Verification items for the finished model (mm, model axes). A direction names the side the tool comes from. Round coordinates to 2 decimals unless told otherwise and drop trailing zeros. Order: outer loops, then holes, each group sorted by start corner. A loop starts at its lowest first (then second) coordinate and runs counter-clockwise, first axis right, second up. Notation, with made-up numbers: (-12, -32) -> (-7, -32) arc R14 ccw to (-7, -20) -> close; hole circle Ø3 at (73.5, 87). An arc over 180 degrees is marked (long way). Return JSON: item names as keys, results as strings. Group by question number.
1) Section check A-A on y = -2.4. State how many separate pieces and enclosed holes the cut face has, plus the area to 3 significant figures.
2) Section check D-D on z = 29. Enter the section's corners in (x, y), plus the area to 3 significant figures.
3) Draft check along Z on faces 5 (the cylindrical face through (-0.065, -1.503, 123.825)), 6 (the flat face through (10, -3.048, 58)), 7 (the flat face through (0, -2, 73)), 8 (the cylindrical face through (-12.038, -1.503, 53.15)). Enter one of: pulls with the +Z half, pulls with the -Z half, needs draft (parallel to the pull), parting line crosses it, or undercut.
4) Section check C-C on z = 51. Enter the section's corners in (x, y), plus the area to 3 significant figures.
5) Scan lines: L1, parallel to Z at x = 44.45, y = -1.05 (3 decimals); L2, parallel to Z at x = -1, y = -1.75; L3, parallel to Z at x = -4.5, y = -1.75. Record each from-to range of solid material in increasing order.
6) Section check B-B on x = -5.5. Enter the section's corners in (y, z), plus the area to 3 significant figures.
7) Depth check by flat-ended pin: pin 1 (5.5 mm diameter, centred on x = 0, z = 114.3, fed in from +Y); pin 2 (1 mm diameter, centred on y = -1.5, z = 98.5, fed in from +X); pin 3 (0.9 mm diameter, centred on y = -2, z = 30, fed in from -X). Enter the tip coordinate at first touch or a pass-through.
8) Tool access check on faces 1 (the flat face through (-0.57, -1.5, 72.92)), 2 (the flat face through (13.134, -1.503, 37.784)), 3 (the flat face through (0, -2, 29)), 4 (the flat face through (10, 0, 58)). Record the directions out of +Z, -Z, +X, -X, +Y, -Y that give a thin tool (end or side, any length) a straight path to the whole face; none if there is none.
```python
from build123d import *

# Parameters (mm, degrees)
F1_DEPTH = 3.048


with BuildPart() as f1:
    # F0 (on Front) → F1 (new body)
    with BuildSketch(Plane.XZ):
        with BuildLine():
            ThreePointArc((15.0989586091, 58.5972381334), (15.6797894265, 61.0180998126), (15.875, 63.5))
            ThreePointArc((15.875, 63.5), (15.843643726, 64.4972855577), (15.7496987737, 65.4906314418))
            Line((15.7496987737, 65.4906314418), (15.0989586091, 58.5972381334))
        make_face()
        with BuildLine():
            Line((15.0989586091, 58.5972381334), (15.7496987737, 65.4906314418))
            ThreePointArc((15.7496987737, 65.4906314418), (10.4979605367, 75.408335298), (0, 79.375))
            Line((0, 79.375), (0, 66.675))
            ThreePointArc((0, 66.675), (2.2450640303, 65.7450640303), (3.175, 63.5))
            ThreePointArc((3.175, 63.5), (2.2450640303, 61.2549359697), (0, 60.325))
            Line((0, 60.325), (0, 47.625))
            ThreePointArc((0, 47.625), (9.3323169783, 50.6577461162), (15.0989586091, 58.5972381334))
        make_face()
        with BuildLine():
            ThreePointArc((0, 79.375), (10.4979605367, 75.408335298), (15.7496987737, 65.4906314418))
            Line((15.7496987737, 65.4906314418), (9.5073556067, 114.8794949239))
            ThreePointArc((9.5073556067, 114.8794949239), (9.5205878798, 114.5898817394), (9.525, 114.3))
            ThreePointArc((9.525, 114.3), (6.7351920908, 107.5648079092), (0, 104.775))
            Line((0, 104.775), (0, 79.375))
        make_face()
        with BuildLine():
            Line((11.2237043258, 17.546057651), (15.0989586091, 58.5972381334))
            ThreePointArc((15.0989586091, 58.5972381334), (9.3323169783, 50.6577461162), (0, 47.625))
            Line((0, 47.625), (0, 9.525))
            ThreePointArc((0, 9.525), (6.7351920908, 6.7351920908), (9.525, 0))
            Line((9.525, 0), (36.5125, 0))
            ThreePointArc((36.5125, 0), (38.9380895153, 5.7116327839), (44.7324052746, 7.9324746146))
            Line((44.7324052746, 7.9324746146), (18.8558582529, 8.853709629))
            ThreePointArc((18.8558582529, 8.853709629), (13.1645636219, 11.5533837704), (11.2237043258, 17.546057651))
        make_face()
        with BuildLine():
            ThreePointArc((-0.9612294652, 79.3458721096), (-0.4808353457, 79.3677163565), (0, 79.375))
            Line((0, 79.375), (0, 104.775))
            ThreePointArc((0, 104.775), (-6.7492648996, 107.5789101839), (-9.5249166577, 114.339845498))
            Line((-9.5249166577, 114.339845498), (-15.7476590945, 65.5067032771))
            ThreePointArc((-15.7476590945, 65.5067032771), (-10.8479208938, 75.0904373205), (-0.9612294652, 79.3458721096))
        make_face()
        with BuildLine():
            ThreePointArc((-0.6240967535, 99.9581825499), (-1.0555795763, 98.8701657595), (-2.1154738069, 98.3735953389))
            ThreePointArc((-2.1154738069, 98.3735953389), (-3.3676139306, 101.0461993403), (-0.6240967535, 99.9581825499))
        make_face(mode=Mode.SUBTRACT)
        with BuildLine():
            ThreePointArc((9.525, 114.3), (9.5205878798, 114.5898817394), (9.5073556067, 114.8794949239))
            ThreePointArc((9.5073556067, 114.8794949239), (-0.2699675413, 123.8211733797), (-9.5249166577, 114.339845498))
            ThreePointArc((-9.5249166577, 114.339845498), (-6.7492648996, 107.5789101839), (0, 104.775))
            ThreePointArc((0, 104.775), (6.7351920908, 107.5648079092), (9.525, 114.3))
        make_face()
        with BuildLine():
            ThreePointArc((3.175, 114.3), (2.2450640303, 112.0549359697), (0, 111.125))
            ThreePointArc((0, 111.125), (-2.2450640303, 116.5450640303), (3.175, 114.3))
        make_face(mode=Mode.SUBTRACT)
        with BuildLine():
            ThreePointArc((-15.0944695401, 58.5834347047), (-9.3264449534, 50.6534810345), (0, 47.625))
            Line((0, 47.625), (0, 60.325))
            ThreePointArc((0, 60.325), (-3.1735432713, 63.4038329309), (-0.192245893, 66.6691744219))
            Line((-0.192245893, 66.6691744219), (-0.9612294652, 79.3458721096))
            ThreePointArc((-0.9612294652, 79.3458721096), (-10.8479208938, 75.0904373205), (-15.7476590945, 65.5067032771))
            Line((-15.7476590945, 65.5067032771), (-15.0944695401, 58.5834347047))
        make_face()
        with BuildLine():
            ThreePointArc((-15.7476590945, 65.5067032771), (-15.8048137164, 62.00886339), (-15.0944695401, 58.5834347047))
            Line((-15.0944695401, 58.5834347047), (-15.7476590945, 65.5067032771))
        make_face()
        with BuildLine():
            ThreePointArc((9.525, 0), (6.7351920908, 6.7351920908), (0, 9.525))
            Line((0, 9.525), (0, 3.175))
            ThreePointArc((0, 3.175), (2.2450640303, 2.2450640303), (3.175, 0))
            Line((3.175, 0), (9.525, 0))
        make_face()
        with BuildLine():
            Line((0, 3.175), (0, 9.525))
            ThreePointArc((0, 9.525), (-9.525, 0), (0, -9.525))
            Line((0, -9.525), (0.6773435479, -9.500885786))
            ThreePointArc((0.6773435479, -9.500885786), (6.9705567315, -6.4912990883), (9.525, 0))
            Line((9.525, 0), (3.175, 0))
            ThreePointArc((3.175, 0), (-2.2450640303, -2.2450640303), (0, 3.175))
        make_face()
        with BuildLine():
            Line((36.5125, 0), (9.525, 0))
            ThreePointArc((9.525, 0), (6.9705567315, -6.4912990883), (0.6773435479, -9.500885786))
            Line((0.6773435479, -9.500885786), (44.7324052746, -7.9324746146))
            ThreePointArc((44.7324052746, -7.9324746146), (38.9380895153, -5.7116327839), (36.5125, 0))
        make_face()
        with BuildLine():
            Line((0.6773435479, -9.500885786), (0, -9.525))
            ThreePointArc((0, -9.525), (0.3388863295, -9.5189695375), (0.6773435479, -9.500885786))
        make_face()
        with BuildLine():
            ThreePointArc((52.3875, 0), (50.1616327839, 5.5119104847), (44.7324052746, 7.9324746146))
            ThreePointArc((44.7324052746, 7.9324746146), (38.9380895153, 5.7116327839), (36.5125, 0))
            ThreePointArc((36.5125, 0), (38.9380895153, -5.7116327839), (44.7324052746, -7.9324746146))
            ThreePointArc((44.7324052746, -7.9324746146), (50.1616327839, -5.5119104847), (52.3875, 0))
        make_face()
        with BuildLine():
            ThreePointArc((47.625, 0), (44.45, -3.175), (41.275, 0))
            ThreePointArc((41.275, 0), (44.45, 3.175), (47.625, 0))
        make_face(mode=Mode.SUBTRACT)
    extrude(amount=F1_DEPTH)


solid = f1.part
```
Check result:
{
 "1": {"separate pieces": "1", "enclosed holes": "5", "area": "3,240 mm^2"},
 "2": {"outline": "(0, -3.05) -> (12.3, -3.05) -> (12.3, 0) -> (0, 0) -> close", "area": "37.5 mm^2"},
 "3": {"face 5": "pulls with the +Z half", "face 6": "needs draft", "face 7": "undercut", "face 8": "undercut"},
 "4": {"outline": "(-9.79, -3.05) -> (14.38, -3.05) -> (14.38, 0) -> (-9.79, 0) -> close", "area": "73.7 mm^2"},
 "5": {"L1": "-7.943 to -3.175, 3.175 to 7.943", "L2": "-9.47 to -3.01, 3.01 to 9.47, 47.66 to 60.49, 66.51 to 98.93, 100.98 to 111.29, 117.31 to 123.77", "L3": "-8.39 to 8.39, 48.28 to 122.69"},
 "6": {"outline": "(-3.05, -7.78) -> (0, -7.78) -> (0, 7.78) -> (-3.05, 7.78) -> close; (-3.05, 48.61) -> (0, 48.61) -> (0, 122.08) -> (-3.05, 122.08) -> close", "area": "271 mm^2"},
 "7": {"pin 1": "through", "pin 2": "x = 11.64", "pin 3": "x = 0"},
 "8": {"face 1": "+Y, -Y", "face 2": "+X, +Y, -Y", "face 3": "-X, +Y, -Y", "face 4": "+Z, -Z, +X, -X, +Y"}
}
